Geometry check sheet. Reference: the model listing, model coordinates, mm. Coordinates: 2 decimals unless noted, no trailing zeros. Loops run counter-clockwise (first coordinate to the right, second up) from the corner with the lowest first, then second, coordinate; pieces in that order, holes last. Notation, with made-up numbers: (50.25, 1) -> (84.25, 1) arc R22 ccw to (84.25, 8) -> close; hole circle Ø10 at (64.25, -8). An arc over 180 degrees is marked (long way). Answer as a JSON object with one key per item and string values.
from build123d import *

# Parameters (mm, degrees)
SKETCH1_R           = 5
BOSS_EXTRUDE1_DEPTH = 1.5
CHAMFER1_SIZE       = 0.5


with BuildPart() as part:
    # Sketch1 → Boss-Extrude1 (new body, symmetric)
    with BuildSketch(Plane(origin=(0, 0, 0), x_dir=(1, 0, 0), z_dir=(0, 1, 0))):
        Polygon((8.082903769, 0), (4.041451884, 7), (-4.041451884, 7), (-8.082903769, 0), (-4.041451884, -7), (4.041451884, -7), align=None)
        Circle(SKETCH1_R, mode=Mode.SUBTRACT)
    extrude(amount=BOSS_EXTRUDE1_DEPTH, both=True)

    # Sketch2 → Cut-Revolve1 (revolve, cut)
    with BuildSketch(Plane.XY):
        Polygon((-8.082903769, 1.5), (-6.582903769, 1.5), (-8.082903769, 0.75), align=None)
        Polygon((-8.082903769, -0.75), (-8.082903769, -1.5), (-6.582903769, -1.5), align=None)
    revolve(axis=Axis((0, -1000, 0), (0, 1, 0)), mode=Mode.SUBTRACT)

    # Chamfer1
    chamfer1_edges = [part.edges().sort_by_distance(p)[0] for p in [
        (-5, -1.5, 0),
        (-5, 1.5, 0),
    ]]
    chamfer(chamfer1_edges, length=CHAMFER1_SIZE)


solid = part.part
1. Section check B-B, the plane y = -0.1. Record the boundary of the cut face in (x, z).
Evaluation:
{"outline": "(-8.08, 0) -> (-4.04, -7) -> (4.04, -7) -> (8.08, 0) -> (4.04, 7) -> (-4.04, 7) -> close; hole circle Ø10 at (0, 0)"}
2. Section check A-A, the plane x = 0. Record the boundary of the cut face in (y, z).
Evaluation:
{"outline": "(-1.5, -6.58) -> (-1.29, -7) -> (1.29, -7) -> (1.5, -6.58) -> (1.5, -5.5) -> (1, -5) -> (-1, -5) -> (-1.5, -5.5) -> close; (-1.5, 5.5) -> (-1, 5) -> (1, 5) -> (1.5, 5.5) -> (1.5, 6.58) -> (1.29, 7) -> (-1.29, 7) -> (-1.5, 6.58) -> close"}
3. Depth check by flat-ended pin: P1, Ø1.5, axis at y = 0, z = 1.5, coming from the -X side; P2, Ø5, axis at x = 5.5, z = 4.5, coming from the -Y side; P3, Ø1.5, axis at y = -0.5, z = -3.5, coming from the +X side. Enter the tip coordinate at first touch or a pass-through.
Evaluation:
{"P1": "stops at x = -7.65", "P2": "stops at y = -1.5", "P3": "stops at x = 6.5"}
4. Thickness scan on probe 1 along Z at (x, y) = (0, 0.4); probe 2 along Z at (x, y) = (4.25, -0.65); probe 3 along X at (y, z) = (-0.25, -1.5). Record the ranges inside material, lowest first. Write a range as from..to.
Evaluation:
{"probe 1": "z = -7..-5, 5..7", "probe 2": "z = -6.64..-2.63, 2.63..6.64", "probe 3": "x = -7.22..-4.77, 4.77..7.22"}
5. Mould release check, pull along Z, two halves, no side actions. Record for faces 1 (the face through (0, 0, -7)), 2 (the face through (-1.08, -0.01, 4.88)), 3 (the face through (-4, 1.5, 4)): released by +Z, released by -Z, zero draft, split by the parting line, or undercut.
Evaluation:
{"face 1": "released by -Z", "face 2": "undercut", "face 3": "zero draft"}
